```python
from build123d import *

# Parameters (mm, degrees)
SKETCH1_R                                       = 15.875
BOSS_EXTRUDE1_DEPTH                             = 3.175
CSK_FOR_M3_FLAT_HEAD_MACHINE_SCREW1_D           = 3.4
CSK_FOR_M3_FLAT_HEAD_MACHINE_SCREW1_CSINK_D     = 6.3
CSK_FOR_M3_FLAT_HEAD_MACHINE_SCREW1_CSINK_ANGLE = 90
F_6_32_TAPPED_HOLE1_D                           = 2.7051


with BuildPart() as part:
    # Sketch1 → Boss-Extrude1 (new body)
    with BuildSketch(Plane.XY):
        Circle(SKETCH1_R)
    extrude(amount=BOSS_EXTRUDE1_DEPTH)

    # CSK for M3 Flat Head Machine Screw1 (through all)
    with Locations(Plane.XY.offset(3.175)):
        with Locations((0, 9.5), (0, -9.5), (12.5, 0), (-12.5, 0)):
            CounterSinkHole(CSK_FOR_M3_FLAT_HEAD_MACHINE_SCREW1_D / 2, CSK_FOR_M3_FLAT_HEAD_MACHINE_SCREW1_CSINK_D / 2, counter_sink_angle=CSK_FOR_M3_FLAT_HEAD_MACHINE_SCREW1_CSINK_ANGLE)

    # #6-32 Tapped Hole1 (through all)
    with Locations(Plane.XY.offset(3.175)):
        with Locations((-6.914797213, 6.914797213), (6.914797213, 6.914797213), (6.914797213, -6.914797213), (-6.914797213, -6.914797213)):
            Hole(F_6_32_TAPPED_HOLE1_D / 2)


solid = part.part
```
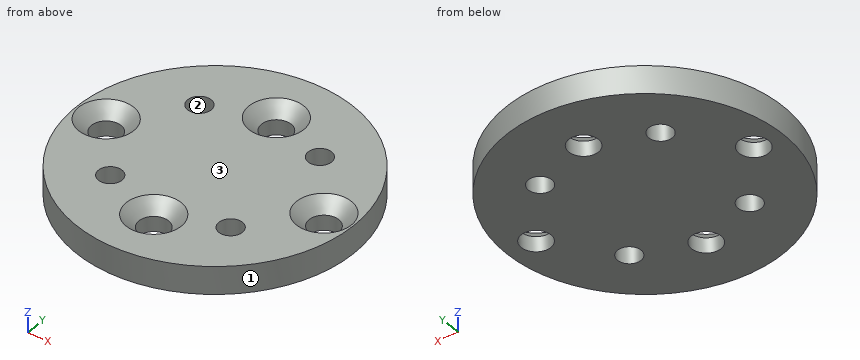
Geometry check sheet. Reference: the model listing, model coordinates, mm. Face numbers are marked on the shaded views. Round coordinates to 2 decimals unless told otherwise and drop trailing zeros. Order: outer loops, then holes, each group sorted by start corner. A loop starts at its lowest first (then second) coordinate and runs counter-clockwise, first axis right, second up. Notation, with made-up numbers: (-20, -4) -> (-13, -4) arc R8 cw to (-13, 6) -> close; hole circle Ø9 at (15, 26.25). An arc over 180 degrees is marked (long way). Return JSON: item names as keys, results as strings. Group by question number.
Q1. Section check D-D, the plane x = -12.5. Record the boundary of the cut face in (y, z) (3 decimals).
Q2. Section check A-A, the plane x = 0. Record the boundary of the cut face in (y, z) (3 decimals).
Q3. Release check for a two-part mould opening along X. For the marked faces 1, 2 and 3 record: released by +X, released by -X, zero draft, split by the parting line, or undercut.
Q4. Material ranges on probe 1 along Y at (x, z) = (0, 0.4) (3 decimals); probe 2 along X at (y, z) = (-6.5, 0.5); probe 3 along X at (y, z) = (-8, 2.65), recorded low to high. Write a range as from..to.
Q5. Section check C-C, the plane z = 2.65. Count the separate pieces of the cut face and the enclosed holes in it, plus the area to 3 significant figures.
Q6. Gauge pin test, flat ends, axial feed: pin 1 (1.6 mm diameter, centred on x = 6.91, y = -6.91, fed in from -Z); pin 2 (4.5 mm diameter, centred on x = -12.5, y = 0, fed in from +Z) (3 decimals). Record the tip position at first contact, or that the pin passes through.
Q7. Section check B-B, the plane y = 0. Record the boundary of the cut face in (x, z) (3 decimals), plus the area to 3 significant figures.
Numbers:
{
 "1": {"outline": "(-9.786, 0) -> (-1.7, 0) -> (-1.7, 1.725) -> (-3.15, 3.175) -> (-9.786, 3.175) -> close; (1.7, 0) -> (9.786, 0) -> (9.786, 3.175) -> (3.15, 3.175) -> (1.7, 1.725) -> close"},
 "2": {"outline": "(-15.875, 0) -> (-11.2, 0) -> (-11.2, 1.725) -> (-12.65, 3.175) -> (-15.875, 3.175) -> close; (-7.8, 0) -> (7.8, 0) -> (7.8, 1.725) -> (6.35, 3.175) -> (-6.35, 3.175) -> (-7.8, 1.725) -> close; (11.2, 0) -> (15.875, 0) -> (15.875, 3.175) -> (12.65, 3.175) -> (11.2, 1.725) -> close"},
 "3": {"face 1": "split by the parting line", "face 2": "undercut", "face 3": "zero draft"},
 "4": {"probe 1": "-15.875..-11.2, -7.8..7.8, 11.2..15.875", "probe 2": "-14.48..-8.2, -5.63..5.63, 8.2..14.48", "probe 3": "-13.71..-7.72, -6.11..-2.15, 2.15..6.11, 7.72..13.71"},
 "5": {"separate pieces": "1", "enclosed holes": "8", "area": "682 mm^2"},
 "6": {"pin 1": "through", "pin 2": "z = 2.275"},
 "7": {"outline": "(-15.875, 0) -> (-14.2, 0) -> (-14.2, 1.725) -> (-15.65, 3.175) -> (-15.875, 3.175) -> close; (-10.8, 0) -> (10.8, 0) -> (10.8, 1.725) -> (9.35, 3.175) -> (-9.35, 3.175) -> (-10.8, 1.725) -> close; (14.2, 0) -> (15.875, 0) -> (15.875, 3.175) -> (15.65, 3.175) -> (14.2, 1.725) -> close", "area": "75.0 mm^2"}
}
